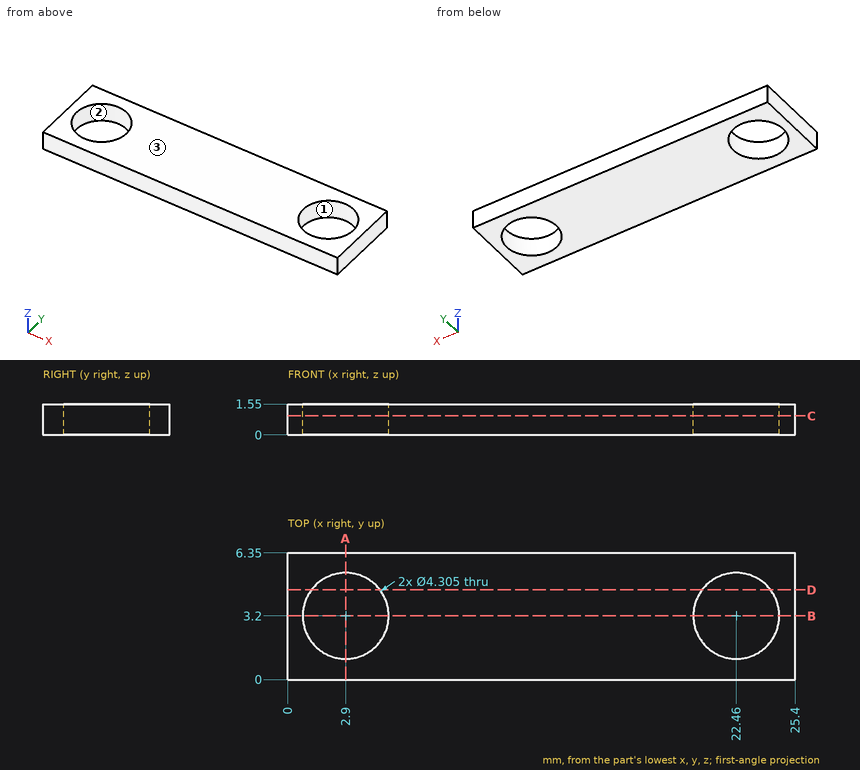
Here's the drawing with two shaded views (mm, measured from the low corner). I have some questions. Give positions to 0.01 mm unless a question says otherwise; leave off trailing zeros. Order: outer loops, then holes, each group sorted by start corner. A loop starts at its lowest first (then second) coordinate and runs counter-clockwise, first axis right, second up. Notation, with made-up numbers: (83.25, 38.5) - (141.25, 38.5) arc R11 cw to (141.25, 49.5) - close; hole circle Ø2 at (-1.5, -37.5). An arc over 180 degrees is marked (long way). Write each question's results on one line, items separated by ' | '.
1) Suppose I cut it at D-D, the plane y = 4.5. Write out the boundary of the cut face in (x, z).
Final values:
outline: (0, 0) - (1.18, 0) - (1.18, 1.55) - (0, 1.55) - close; (4.62, 0) - (20.74, 0) - (20.74, 1.55) - (4.62, 1.55) - close; (24.18, 0) - (25.4, 0) - (25.4, 1.55) - (24.18, 1.55) - close
2) Please list where these lines run through material, in increasing order: line 1 along X through (y, z) = (3.5, 0.65); line 2 along X through (y, z) = (3.75, 0.75); line 3 along Y through (x, z) = (2.9, 0.7). Write a range as [from, to].
Final values:
line 1: x = [0, 0.77], [5.03, 20.33], [24.59, 25.4] | line 2: x = [0, 0.82], [4.98, 20.38], [24.54, 25.4] | line 3: y = [0, 1.05], [5.35, 6.35]
3) Suppose I cut it at B-B, the plane y = 3.2. Write out the boundary of the cut face in (x, z), then the cut area to 3 significant figures.
Final values:
outline: (0, 0) - (0.75, 0) - (0.75, 1.55) - (0, 1.55) - close; (5.05, 0) - (20.31, 0) - (20.31, 1.55) - (5.05, 1.55) - close; (24.61, 0) - (25.4, 0) - (25.4, 1.55) - (24.61, 1.55) - close | area: 26.0 mm^2
4) If we mould it in two halves opening along Y, with no side actions, what happens to the marked faces 1, 2 and 3? For each: pulls with the +Y half, pulls with the -Y half, needs draft (parallel to the pull), parting line crosses it, or undercut.
Final values:
face 1: undercut | face 2: undercut | face 3: needs draft
5) Suppose I cut it at C-C, the plane z = 0.95. Give the number of separate pieces and of enclosed holes in the cut face, then the cut area to 3 significant figures.
Final values:
separate pieces: 1 | enclosed holes: 2 | area: 132 mm^2
6) Suppose I cut it at A-A, the plane x = 2.9. Write out the boundary of the cut face in (y, z).
Final values:
outline: (0, 0) - (1.05, 0) - (1.05, 1.55) - (0, 1.55) - close; (5.35, 0) - (6.35, 0) - (6.35, 1.55) - (5.35, 1.55) - close
